Check sheet for the modelled part. Datum: model origin and axes. Units: mm. A direction names the side the tool comes from. Round coordinates to 2 decimals unless told otherwise and drop trailing zeros.
```python
from build123d import *

# Parameters (mm, degrees)
BOSS_EXTRUDE1_DEPTH          = 0.381
SKETCH2_R                    = 1.5
CUT_EXTRUDE1_DEPTH           = 0.127
SKETCH17_R                   = 1.5
CUT_EXTRUDE9_DEPTH           = 0.2
HEART_SYM_CUT_EXTRUDE6_DEPTH = 0.005
BATT_SYM_CUT_EXTRUDE7_DEPTH  = 0.005
COMM_SYMCUT_EXTRUDE9_DEPTH   = 0.1


with BuildPart() as part:
    # Sketch1 → Boss-Extrude1 (new body)
    with BuildSketch(Plane.XY):
        with BuildLine():
            Line((2.14, 0), (59.46, 0))
            ThreePointArc((59.46, 0), (60.973208512, 0.626791488), (61.6, 2.14))
            Line((61.6, 2.14), (61.6, 23.26))
            ThreePointArc((61.6, 23.26), (60.973208512, 24.773208512), (59.46, 25.4))
            Line((59.46, 25.4), (2.14, 25.4))
            ThreePointArc((2.14, 25.4), (0.626791488, 24.773208512), (0, 23.26))
            Line((0, 23.26), (0, 2.14))
            ThreePointArc((0, 2.14), (0.626791488, 0.626791488), (2.14, 0))
        make_face()
    extrude(amount=BOSS_EXTRUDE1_DEPTH)

    # Sketch2 → Cut-Extrude1 (cut)
    with BuildSketch(Plane.XY.offset(0.381)):
        with Locations((58.125, 18.8976)):
            Circle(SKETCH2_R)
        with Locations((58.125, 7.3914)):
            Circle(SKETCH2_R)
    extrude(amount=-CUT_EXTRUDE1_DEPTH, mode=Mode.SUBTRACT)

    # Sketch17 → Cut-Extrude9 (cut)
    with BuildSketch(Plane.XY.offset(0.381)):
        with Locations((3.475, 18.8976)):
            Circle(SKETCH17_R)
    extrude(amount=-CUT_EXTRUDE9_DEPTH, mode=Mode.SUBTRACT)

    # Sketch10 → Heart Sym Cut-Extrude6 (cut)
    with BuildSketch(Plane.XY.offset(0.381)):
        with BuildLine():
            ThreePointArc((51.625, 19.4976), (50.125, 20.9976), (48.625, 19.4976))
            ThreePointArc((48.625, 19.4976), (49.450765386, 16.899523789), (51.625, 15.254959313))
            ThreePointArc((51.625, 15.254959313), (53.799234614, 16.899523789), (54.625, 19.4976))
            ThreePointArc((54.625, 19.4976), (53.125, 20.9976), (51.625, 19.4976))
        make_face()
    extrude(amount=-HEART_SYM_CUT_EXTRUDE6_DEPTH, mode=Mode.SUBTRACT)

    # Sketch11 → Batt Sym Cut-Extrude7 (cut)
    with BuildSketch(Plane.XY.offset(0.381)):
        with BuildLine():
            Line((7.175, 20.3976), (7.775, 20.3976))
            Line((7.775, 20.3976), (7.775, 20.6976))
            ThreePointArc((7.775, 20.6976), (7.833578644, 20.839021356), (7.975, 20.8976))
            Line((7.975, 20.8976), (8.975, 20.8976))
            ThreePointArc((8.975, 20.8976), (9.116421356, 20.839021356), (9.175, 20.6976))
            Line((9.175, 20.6976), (9.175, 20.3976))
            Line((9.175, 20.3976), (9.775, 20.3976))
            ThreePointArc((9.775, 20.3976), (9.916421356, 20.339021356), (9.975, 20.1976))
            Line((9.975, 20.1976), (9.975, 16.0976))
            ThreePointArc((9.975, 16.0976), (9.916421356, 15.956178644), (9.775, 15.8976))
            Line((9.775, 15.8976), (7.175, 15.8976))
            ThreePointArc((7.175, 15.8976), (7.033578644, 15.956178644), (6.975, 16.0976))
            Line((6.975, 16.0976), (6.975, 20.1976))
            ThreePointArc((6.975, 20.1976), (7.033578644, 20.339021356), (7.175, 20.3976))
        make_face()
    extrude(amount=-BATT_SYM_CUT_EXTRUDE7_DEPTH, mode=Mode.SUBTRACT)

    # Sketch13 → Comm SymCut-Extrude9 (cut)
    with BuildSketch(Plane.XY.offset(0.381)):
        Polygon((53.810786438, 7.805613562), (53.174390335, 7.169217459), (53.502207794, 6.8414), (51.225, 6.8414), (51.225, 5.9414), (53.502207794, 5.9414), (53.174390335, 5.613582541), (53.810786438, 4.977186438), (55.225, 6.3914), align=None)
        Polygon((49.847792206, 7.9414), (50.175609665, 7.613582541), (49.539213562, 6.977186438), (48.125, 8.3914), (49.539213562, 9.805613562), (50.175609665, 9.169217459), (49.847792206, 8.8414), (52.125, 8.8414), (52.125, 7.9414), align=None)
    extrude(amount=-COMM_SYMCUT_EXTRUDE9_DEPTH, mode=Mode.SUBTRACT)


solid = part.part
```
Item 1: Access from +Z, -Z, +X, -X, +Y, -Y to the whole of each face (thin tool, end or side, straight path). Record for faces 1 (the flat face through (3, 19, 0.181)), 2 (the cylindrical face through (0.644, 24.79, 0.188)).
Answer:
face 1: +Z
face 2: +Z, -Z, -X, +Y
Item 2: Release check for a two-part mould opening along Y. For faces 3 (the cylindrical face through (60.956, 0.61, 0.188)), 4 (the flat face through (30, 13, 0.381)), 5 (the cylindrical face through (60.99, 24.756, 0.188)), 6 (the flat face through (58, 7, 0.254)) record: released by +Y, released by -Y, zero draft, split by the parting line, or undercut.
Answer:
face 3: released by -Y
face 4: zero draft
face 5: released by +Y
face 6: undercut
Item 3: Go/stop test with flat-tipped pins: P1, Ø2.5, axis at x = 58.12, y = 18.9, coming from the +Z side; P2, Ø0.9, axis at x = 4, y = 18.5, coming from the +Z side. Record where each tip stops, or that it passes through.
Answer:
P1: stops at z = 0.25
P2: stops at z = 0.18
